Can you work these out from the model? Positions are in its coordinate system, mm. A direction names the side the tool comes from. Give positions to 0.01 mm unless a question says otherwise; leave off trailing zeros. Loops run counter-clockwise (first coordinate to the right, second up) from the corner with the lowest first, then second, coordinate; pieces in that order, holes last. Notation, with made-up numbers: (59.5, -34.5) - (97.5, -34.5) arc R18 cw to (97.5, -14.5) - close; hole circle Ø3 at (23.25, 19.5). An arc over 180 degrees is marked (long way). Answer as a JSON object with one key per item and string values. Group by question number.
Item 1: Please list where these lines run through material, in increasing order: L1, parallel to Z at x = 0, y = 5.5; L2, parallel to X at y = 8, z = 0; L3, parallel to Y at x = -5, z = -9.5.
Item 2: Suppose I cut it at C-C on y = 1.5. Write out the boundary of the cut face in (x, z).
Item 3: Thinking about a two-plate mould opening in X: for faces 1 (the cylindrical face through (9.7, 0.99, -6.18)), 2 (the flat face through (-1.45, 10, 5)), 3 (the flat face through (0, 0, -5)), which applies, pulls with the +X half, pulls with the -X half, needs draft (parallel to the pull), parting line crosses it, or undercut?
Item 4: Which directions (+Z, -Z, +X, -X, +Y, -Y) give clear straight access to the entire face, cutting with the end or side of a thin tool? Please do faces 4 (the flat face through (0, 10, 6)), 5 (the flat face through (-2, 20, -4)), 6 (the flat face through (9, 2, 4)).
Item 5: Suppose I cut it at D-D on x = 10. Write out the boundary of the cut face in (y, z).
Item 6: Suppose I cut it at B-B on z = 0. Write out the boundary of the cut face in (x, y).
Item 7: Will these pins go through, and if not, where does the flat tip stop? pin 1 (6 mm diameter, centred on x = 8.5, y = 14, fed in from +Z); pin 2 (1 mm diameter, centred on y = 14.5, z = -8.5, fed in from -X); pin 3 (3 mm diameter, centred on x = 0, y = 13, fed in from -Z); pin 4 (7 mm diameter, centred on x = 0, z = 0, fed in from -Y).
Item 8: Suppose I cut it at A-A on x = 0. Write out the boundary of the cut face in (y, z), and give its area (3 significant figures).
from build123d import *

# Parameters (mm, degrees)
SKETCH1_R           = 9.55
BOSS_EXTRUDE1_DEPTH = 20
CHAMFER1_SIZE       = 1.5
SKETCH2_R           = 11.5
SKETCH2_R_2         = 9.55
BOSS_EXTRUDE2_DEPTH = 2


with BuildPart() as part:
    # Sketch1 → Boss-Extrude1 (new body)
    with BuildSketch(Plane(origin=(0, 0, 0), x_dir=(1, 0, 0), z_dir=(0, 1, 0))):
        with Locations(Location((0, 0, 0), (0, 0, 270))):
            Circle(SKETCH1_R)
        with BuildLine():
            Line((-1.45, -6), (1.45, -6))
            Line((1.45, -6), (1.45, -3.727935085))
            ThreePointArc((1.45, -3.727935085), (0, 4), (-1.45, -3.727935085))
            Line((-1.45, -3.727935085), (-1.45, -6))
        make_face(mode=Mode.SUBTRACT)
    extrude(amount=BOSS_EXTRUDE1_DEPTH)

    # Chamfer1
    chamfer1_edges = [part.edges().sort_by_distance(p)[0] for p in [
        (0, 20, -9.55),
    ]]
    chamfer(chamfer1_edges, length=CHAMFER1_SIZE)

    # Sketch2 → Boss-Extrude2 (add)
    with BuildSketch(Plane.XZ):
        with Locations(Location((0, 0, 0), (0, 0, 270))):
            Circle(SKETCH2_R)
        with Locations(Location((0, 0, 0), (0, 0, 270))):
            Circle(SKETCH2_R_2, mode=Mode.SUBTRACT)
    extrude(amount=-BOSS_EXTRUDE2_DEPTH)


solid = part.part
Worked out:
{
 "1": {"L1": "z = -9.55 to -4, 6 to 9.55", "L2": "x = -9.55 to -4, 4 to 9.55", "L3": "y = 0 to 2"},
 "2": {"outline": "circle Ø23 at (0, 0); hole (-1.45, 3.73) arc R4 ccw (long way) to (1.45, 3.73) - (1.45, 6) - (-1.45, 6) - close"},
 "3": {"face 1": "parting line crosses it", "face 2": "undercut", "face 3": "needs draft"},
 "4": {"face 4": "+Y, -Y", "face 5": "+Z, -Z, +X, -X, +Y", "face 6": "+Y"},
 "5": {"outline": "(0, -5.68) - (2, -5.68) - (2, 5.68) - (0, 5.68) - close"},
 "6": {"outline": "(-11.5, 0) - (-4, 0) - (-4, 20) - (-8.05, 20) - (-9.55, 18.5) - (-9.55, 2) - (-11.5, 2) - close; (4, 0) - (11.5, 0) - (11.5, 2) - (9.55, 2) - (9.55, 18.5) - (8.05, 20) - (4, 20) - close"},
 "7": {"pin 1": "stops at z = 7.81", "pin 2": "stops at x = -5.22", "pin 3": "stops at z = -9.55", "pin 4": "passes through"},
 "8": {"outline": "(0, -11.5) - (2, -11.5) - (2, -9.55) - (18.5, -9.55) - (20, -8.05) - (20, -4) - (0, -4) - close; (0, 6) - (20, 6) - (20, 8.05) - (18.5, 9.55) - (2, 9.55) - (2, 11.5) - (0, 11.5) - close", "area": "188 mm2"}
}
